Can you work these out from the drawing? Everything is in mm from the part's minimum corner. A direction names the side the tool comes from. Give positions to 0.01 mm unless a question says otherwise; leave off trailing zeros. Loops run counter-clockwise (first coordinate to the right, second up) from the corner with the lowest first, then second, coordinate; pieces in that order, holes last.
Q1. If we section it at C-C (z = 3.75): Please give me the cut outline in (x, y).
Q2. If we section it at D-D (z = 13): Please give me the cut outline in (x, y), plus the area to 3 significant figures.
Q3. Will these pins go through, and if not, where does the flat tip stop? P1, Ø4, axis at y = 12, z = 11.5, coming from the +X side; P2, Ø8, axis at x = 14.5, y = 9.5, coming from the -Z side; P3, Ø1, axis at y = 11.5, z = 8, coming from the -X side; P4, Ø2, axis at y = 13, z = 6, coming from the +X side.
Q4. For the marked faces 1 and 2, which set-ups out of +Z, -Z, +X, -X, +Y, -Y let a thin tool reach every point of the face, with its end or its side?
Q5. I need wall thicknesses on line 1 (Z direction, x = 11, y = 14); line 2 (Y direction, x = 2, z = 1.25) (1 decimal); line 3 (Y direction, x = 11.25, z = 10.25) (1 decimal). Which ranges of each line are inside material? Lowest first, please.
Q6. If we section it at A-A (y = 9): Please give me the cut outline in (x, z).
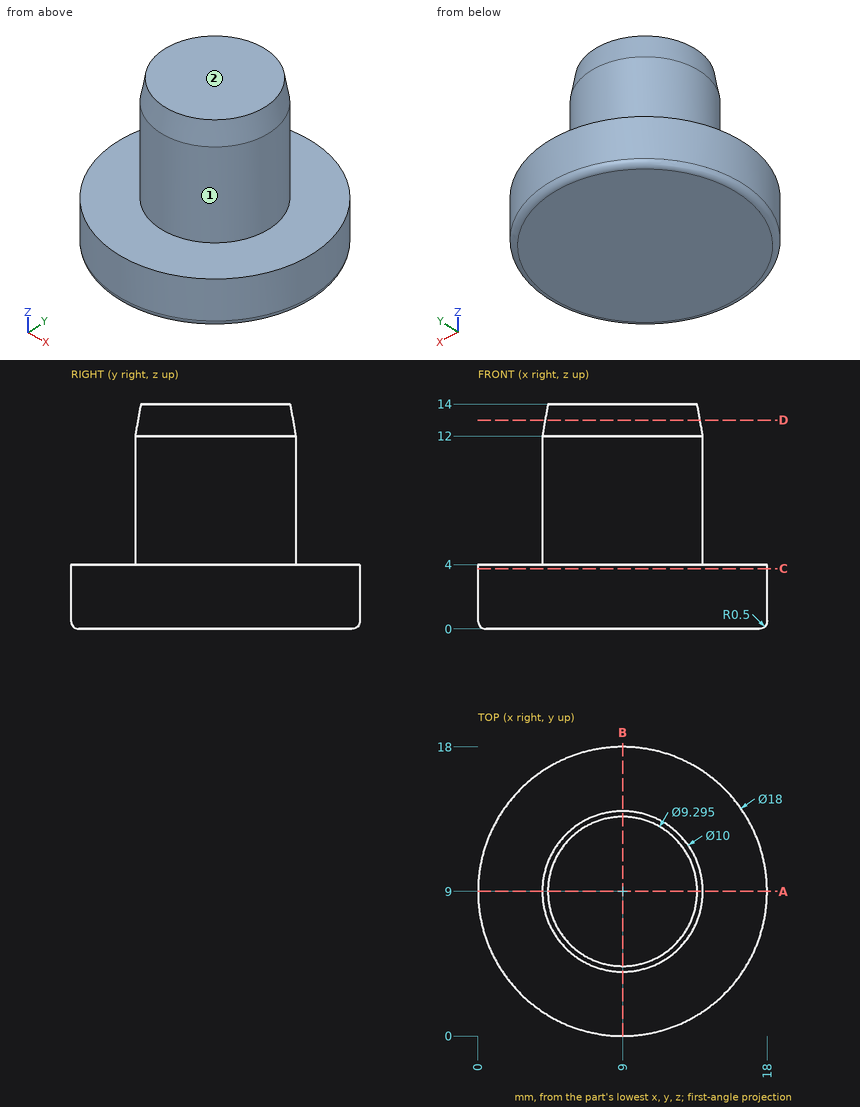
Check sheet entries:
1. outline: circle Ø18 at (9, 9)
2. outline: circle Ø9.65 at (9, 9)
2. area: 73.1 mm2
3. P1: stops at x = 13.9
3. P2: stops at z = 0
3. P3: stops at x = 4.42
3. P4: stops at x = 13
4. face 1: +Z
4. face 2: +Z, +X, -X, +Y, -Y
5. line 1: z = 0 to 4
5. line 2: y = 3.3 to 14.7
5. line 3: y = 4.5 to 13.5
6. outline: (0, 0.5) arc R0.5 ccw to (0.5, 0) - (17.5, 0) arc R0.5 ccw to (18, 0.5) - (18, 4) - (14, 4) - (14, 12) - (13.65, 14) - (4.35, 14) - (4, 12) - (4, 4) - (0, 4) - close
